Here's how the part is built. I have some questions about the finished solid (model axes, mm). A direction names the side the tool comes from. Give positions to 0.01 mm unless a question says otherwise; leave off trailing zeros. Write each loop counter-clockwise with the first axis right and the second up, starting at its lowest first coordinate (ties: lowest second). Pieces come first, ordered by that corner, then holes. Notation, with made-up numbers: (54.25, 18.5) - (91.25, 18.5) arc R22 ccw to (91.25, 49.5) - close; hole circle Ø4 at (-38.5, -22.75). An arc over 180 degrees is marked (long way). Use one line per item in the form item = value. Start each with the question number.
from build123d import *

# Parameters (mm, degrees)
F1_DEPTH = 44.45
F2_R     = 19.05


with BuildPart() as f1:
    # F0 (on Front) → F1 (new body)
    with BuildSketch(Plane.XZ):
        with BuildLine():
            Line((-39.009379, 65.874033), (-39.009379, 63.842033))
            Line((-39.009379, 63.842033), (2.900621, 63.842033))
            ThreePointArc((2.900621, 63.842033), (6.492723, 62.354135), (7.980621, 58.762033))
            Line((7.980621, 58.762033), (7.980621, 52.412033))
            ThreePointArc((7.980621, 52.412033), (6.492723, 48.81993), (2.900621, 47.332033))
            Line((2.900621, 47.332033), (1.630621, 47.332033))
            ThreePointArc((1.630621, 47.332033), (-1.961481, 45.844135), (-3.449379, 42.252033))
            Line((-3.449379, 42.252033), (-3.449379, -110.147967))
            Line((-3.449379, -110.147967), (-1.417379, -110.147967))
            Line((-1.417379, -110.147967), (-1.417379, 42.252033))
            ThreePointArc((-1.417379, 42.252033), (-0.52464, 44.407294), (1.630621, 45.300033))
            Line((1.630621, 45.300033), (2.900621, 45.300033))
            ThreePointArc((2.900621, 45.300033), (7.929564, 47.383089), (10.012621, 52.412033))
            Line((10.012621, 52.412033), (10.012621, 58.762033))
            ThreePointArc((10.012621, 58.762033), (7.929564, 63.790976), (2.900621, 65.874033))
            Line((2.900621, 65.874033), (-39.009379, 65.874033))
        make_face()
    extrude(amount=F1_DEPTH)

    # F2
    f2_edges = [f1.edges().sort_by_distance(p)[0] for p in [
        (-39.009379, 0, 64.858033),
        (-39.009379, -44.45, 64.858033),
    ]]
    fillet(f2_edges, radius=F2_R)


solid = f1.part
1. I want a section at C-C, the plane x = -17. List the corners of the cut face in (y, z) for me.
2. For P1, Ø1, axis at x = 1, y = -30, coming from the -Z side; P2, Ø1.5, axis at x = -10, y = -17, coming from the -Z side; P3, Ø3, axis at y = -17, z = 55.5, coming from the -X side, each with a flat end and sliding along its axis, tell me the tip position at first contact or that it passes through.
3. I want a section at D-D, the plane y = -5. List the corners of the cut face in (x, z) for me, then the cut area to 3 significant figures.
4. For faces 4 (the face through (10.013, -22, 56)), 5 (the face through (-3.449, -22, -33)), 6 (the face through (7.981, -22, 56)), which set-ups out of +Z, -Z, +X, -X, +Y, -Y let a thin tool reach every point of the face, with its end or its side?
5. We'd pull the mould along Z, two halves only. Please class faces 1 (the face through (-1.417, -22, -35)), 2 (the face through (7.98, -21.91, 63.74)), 3 (the face through (6.453, -21.914, 62.393)): pulls with the +Z half, pulls with the -Z half, needs draft (parallel to the pull), parting line crosses it, or undercut.
6. Please list where these lines run through material, in increasing order: line 1 (X direction, y = -29, z = 58.5); line 2 (X direction, y = -41.5, z = -8); line 3 (Z direction, x = 3, y = -34).
7. I want a section at A-A, the plane y = -23.5. List the corners of the cut face in (x, z) for me, then the cut area to 3 significant figures.
8. I want a section at B-B, the plane z = 38. List the corners of the cut face in (x, y) for me, then the cut area to 3 significant figures.
Result sheet:
q1.outline = (-44.45, 63.84) - (0, 63.84) - (0, 65.87) - (-44.45, 65.87) - close
q2.P1 = 45.08
q2.P2 = 63.84
q2.P3 = 7.98
q3.outline = (-32.82, 63.84) - (2.9, 63.84) arc R5.08 cw to (7.98, 58.76) - (7.98, 52.41) arc R5.08 cw to (2.9, 47.33) - (1.63, 47.33) arc R5.08 ccw to (-3.45, 42.25) - (-3.45, -110.15) - (-1.42, -110.15) - (-1.42, 42.25) arc R3.05 cw to (1.63, 45.3) - (2.9, 45.3) arc R7.11 ccw to (10.01, 52.41) - (10.01, 58.76) arc R7.11 ccw to (2.9, 65.87) - (-32.82, 65.87) - close
q3.area = 450 mm2
q4.face_4 = +Z, -Z, +X, +Y, -Y
q4.face_5 = -Z, -X, +Y, -Y
q4.face_6 = -X, +Y, -Y
q5.face_1 = needs draft
q5.face_2 = pulls with the +Z half
q5.face_3 = undercut
q6.line_1 = 7.98 to 10.01
q6.line_2 = -3.45 to -1.42
q6.line_3 = 45.3 to 47.33, 63.84 to 65.87
q7.outline = (-39.01, 63.84) - (2.9, 63.84) arc R5.08 cw to (7.98, 58.76) - (7.98, 52.41) arc R5.08 cw to (2.9, 47.33) - (1.63, 47.33) arc R5.08 ccw to (-3.45, 42.25) - (-3.45, -110.15) - (-1.42, -110.15) - (-1.42, 42.25) arc R3.05 cw to (1.63, 45.3) - (2.9, 45.3) arc R7.11 ccw to (10.01, 52.41) - (10.01, 58.76) arc R7.11 ccw to (2.9, 65.87) - (-39.01, 65.87) - close
q7.area = 462 mm2
q8.outline = (-3.45, -44.45) - (-1.42, -44.45) - (-1.42, 0) - (-3.45, 0) - close
q8.area = 90.3 mm2
